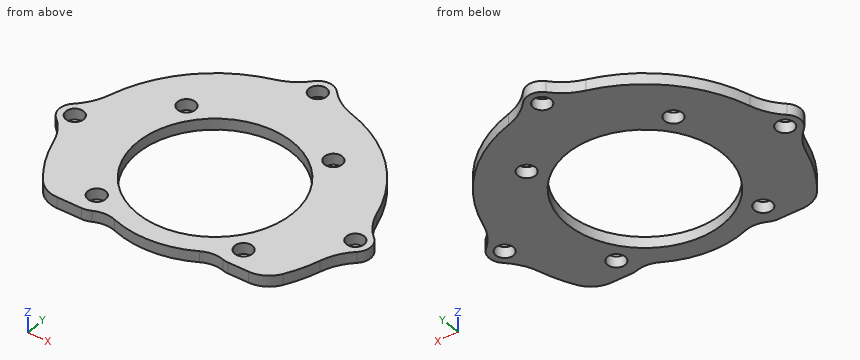
from build123d import *

# Parameters (mm, degrees)
SKETCH1_R           = 25
SKETCH1_R_2         = 3
BOSS_EXTRUDE1_DEPTH = 2
FILLET1_R           = 10
CUT_EXTRUDE1_DEPTH  = 3.0000001
SKETCH4_R           = 1.6
SKETCH4_R_2         = 14
CUT_EXTRUDE2_DEPTH  = 3.0000001
SKETCH6_R           = 1.6
CUT_EXTRUDE3_DEPTH  = 3.0000001
SKETCH7_OUTSIDE_W   = 73.426
SKETCH7_OUTSIDE_H   = 70.426
CUT_EXTRUDE4_DEPTH  = 10
CUT_EXTRUDE5_DEPTH  = 10
FILLET2_R           = 5


with BuildPart() as part:
    # Sketch1 → Boss-Extrude1 (new body)
    with BuildSketch(Plane.XY):
        with Locations((-25, -40.1)):
            Circle(SKETCH1_R)
        with Locations((-50, -40.1)):
            Circle(SKETCH1_R_2)
        with Locations((-50, -40.1)):
            Circle(SKETCH1_R_2)
        with Locations((-25, -40.1)):
            Circle(SKETCH1_R)
        with Locations((0, -40.1)):
            Circle(SKETCH1_R_2)
        with Locations((-25, -40.1)):
            Circle(SKETCH1_R)
        with Locations((-25, -15.1)):
            Circle(SKETCH1_R_2)
        with Locations((-50, -40.1)):
            Circle(SKETCH1_R_2)
        with Locations((-25, -40.1)):
            Circle(SKETCH1_R)
        with Locations((-25, -15.1)):
            Circle(SKETCH1_R_2)
        with Locations((-25, -15.1)):
            Circle(SKETCH1_R_2)
        with Locations((-25, -40.1)):
            Circle(SKETCH1_R)
        with Locations((-25, -40.1)):
            Circle(SKETCH1_R)
        with Locations((0, -40.1)):
            Circle(SKETCH1_R_2)
        with Locations((0, -40.1)):
            Circle(SKETCH1_R_2)
        with Locations((-25, -40.1)):
            Circle(SKETCH1_R)
    extrude(amount=BOSS_EXTRUDE1_DEPTH)

    # Fillet1
    fillet1_edges = [part.edges().sort_by_distance(p)[0] for p in [
        (-49.82, -37.105404869, 1),
        (-27.994595131, -15.28, 1),
        (-22.005404869, -15.28, 1),
        (-0.18, -37.105404869, 1),
        (-0.18, -43.094595131, 1),
        (-49.82, -43.094595131, 1),
    ]]
    fillet(fillet1_edges, radius=FILLET1_R)

    # Sketch3 → Cut-Extrude1 (cut, through all)
    with BuildSketch(Plane.XY.offset(2)):
        with BuildLine():
            ThreePointArc((-37.216735292, -29.767928139), (-37.401620542, -27.65468006), (-39.514868621, -27.83956531))
            ThreePointArc((-39.514868621, -27.83956531), (-39.329983371, -29.952813389), (-37.216735292, -29.767928139))
        make_face()
        with BuildLine():
            ThreePointArc((-35.332071861, -52.316735292), (-37.44531994, -52.501620542), (-37.26043469, -54.614868621))
            ThreePointArc((-37.26043469, -54.614868621), (-35.147186611, -54.429983371), (-35.332071861, -52.316735292))
        make_face()
        with BuildLine():
            ThreePointArc((-12.783264708, -50.432071861), (-12.598379458, -52.54531994), (-10.485131379, -52.36043469))
            ThreePointArc((-10.485131379, -52.36043469), (-10.670016629, -50.247186611), (-12.783264708, -50.432071861))
        make_face()
        with BuildLine():
            ThreePointArc((-14.667928139, -27.883264708), (-12.55468006, -27.698379458), (-12.73956531, -25.585131379))
            ThreePointArc((-12.73956531, -25.585131379), (-14.852813389, -25.770016629), (-14.667928139, -27.883264708))
        make_face()
        with BuildLine():
            ThreePointArc((-35.264995538, -31.48664603), (-33.61335397, -50.364995538), (-14.735004462, -48.71335397))
            ThreePointArc((-14.735004462, -48.71335397), (-16.38664603, -29.835004462), (-35.264995538, -31.48664603))
        make_face()
    extrude(amount=-CUT_EXTRUDE1_DEPTH, mode=Mode.SUBTRACT)

    # Sketch4 → Cut-Extrude2 (cut, through all)
    with BuildSketch(Plane.XY.offset(2)):
        with Locations((-36.296253275, -53.465801956)):
            Circle(SKETCH4_R)
        with Locations((-38.365801956, -28.803746725)):
            Circle(SKETCH4_R)
        with Locations((-13.703746725, -26.734198044)):
            Circle(SKETCH4_R)
        with Locations((-11.634198044, -51.396253275)):
            Circle(SKETCH4_R)
        with Locations((-25, -40.1)):
            Circle(SKETCH4_R_2)
    extrude(amount=-CUT_EXTRUDE2_DEPTH, mode=Mode.SUBTRACT)

    # Sketch6 → Cut-Extrude3 (cut, through all)
    with BuildSketch(Plane.XY.offset(2)):
        with Locations((-50, -40.1)):
            Circle(SKETCH6_R)
        with Locations((-25, -15.1)):
            Circle(SKETCH6_R)
        with Locations((0, -40.1)):
            Circle(SKETCH6_R)
    extrude(amount=-CUT_EXTRUDE3_DEPTH, mode=Mode.SUBTRACT)

    # Sketch7 outside → Cut-Extrude4 (cut)
    with BuildSketch(Plane.XY.offset(2)):
        with Locations((-25, -38.6)):
            Rectangle(SKETCH7_OUTSIDE_W, SKETCH7_OUTSIDE_H)
        with BuildLine():
            ThreePointArc((-31.881324829, -16.325857143), (-42.500892834, -22.599107166), (-48.774142857, -33.218675171))
            ThreePointArc((-48.774142857, -33.218675171), (-49.956443907, -35.846542569), (-51.823461538, -38.041484025))
            ThreePointArc((-51.823461538, -38.041484025), (-52.75, -40.1), (-51.823461538, -42.158515975))
            ThreePointArc((-51.823461538, -42.158515975), (-49.956443907, -44.353457431), (-48.774142857, -46.981324829))
            ThreePointArc((-48.774142857, -46.981324829), (-25, -64.85), (-1.225857143, -46.981324829))
            ThreePointArc((-1.225857143, -46.981324829), (-0.043556093, -44.353457431), (1.823461538, -42.158515975))
            ThreePointArc((1.823461538, -42.158515975), (2.75, -40.1), (1.823461538, -38.041484025))
            ThreePointArc((1.823461538, -38.041484025), (-0.043556093, -35.846542569), (-1.225857143, -33.218675171))
            ThreePointArc((-1.225857143, -33.218675171), (-7.499107166, -22.599107166), (-18.118675171, -16.325857143))
            ThreePointArc((-18.118675171, -16.325857143), (-20.746542569, -15.143556093), (-22.941484025, -13.276538462))
            ThreePointArc((-22.941484025, -13.276538462), (-25, -12.35), (-27.058515975, -13.276538462))
            ThreePointArc((-27.058515975, -13.276538462), (-29.253457431, -15.143556093), (-31.881324829, -16.325857143))
        make_face(mode=Mode.SUBTRACT)
    extrude(amount=-CUT_EXTRUDE4_DEPTH, mode=Mode.SUBTRACT)

    # Sketch8 → Cut-Extrude5 (cut)
    with BuildSketch(Plane.XY.offset(2)):
        with BuildLine():
            ThreePointArc((-33.189286906, -55.565625754), (-34.537253452, -56.777662403), (-36.296253275, -57.215801956))
            Line((-36.296253275, -57.215801956), (-42.877690662, -57.215801956))
            ThreePointArc((-42.877690662, -57.215801956), (-23.637222782, -64.812453101), (-5.348721101, -55.146253275))
            Line((-5.348721101, -55.146253275), (-11.634198044, -55.146253275))
            ThreePointArc((-11.634198044, -55.146253275), (-13.110091293, -54.843605755), (-14.347757645, -53.984514137))
            ThreePointArc((-14.347757645, -53.984514137), (-23.536608094, -57.538706492), (-33.189286906, -55.565625754))
        make_face()
    extrude(amount=-CUT_EXTRUDE5_DEPTH, mode=Mode.SUBTRACT)

    # Fillet2
    fillet2_edges = [part.edges().sort_by_distance(p)[0] for p in [
        (-42.877690662, -57.215801956, 1),
        (-5.348721101, -55.146253275, 1),
        (-14.347757645, -53.984514137, 1),
        (-33.189286906, -55.565625754, 1),
    ]]
    fillet(fillet2_edges, radius=FILLET2_R)


solid = part.part
CAD build for the part. Positions are in the model's coordinates, mm. Give positions to 0.01 mm unless a question says otherwise; leave off trailing zeros. Write each loop counter-clockwise with the first axis right and the second up, starting at its lowest first coordinate (ties: lowest second). Pieces come first, ordered by that corner, then holes. Notation, with made-up numbers: (-23.5, 70.5) - (8.5, 70.5) arc R28 ccw to (8.5, 93.5) - close; hole circle Ø4 at (62, 41). An arc over 180 degrees is marked (long way). Put each result on its own line as item: value.
(1) Wall check: L1, parallel to Y at x = -25, z = 0.9; L2, parallel to Y at x = -24, z = 1.9; L3, parallel to X at y = -49.5, z = 0.7. Give the ranges that are in metal, low to high.
Working result:
L1: -57.6 to -54.1, -26.1 to -16.7, -13.5 to -12.35
L2: -57.57 to -54.06, -26.14 to -16.35, -13.85 to -12.54
L3: -47.9 to -35.37, -14.63 to -2.1
(2) Saw through at C-C (x = 0). List the corners of the cut face in (y, z), then the cut area to 3 significant figures.
Working result:
outline: (-44.29, 0) - (-41.7, 0) - (-41.7, 2) - (-44.29, 2) - close; (-38.5, 0) - (-35.91, 0) - (-35.91, 2) - (-38.5, 2) - close
area: 10.3 mm^2
(3) Saw through at D-D (y = -15.1). List the corners of the cut face in (x, z), then the cut area to 3 significant figures.
Working result:
outline: (-29.19, 0) - (-26.6, 0) - (-26.6, 2) - (-29.19, 2) - close; (-23.4, 0) - (-20.81, 0) - (-20.81, 2) - (-23.4, 2) - close
area: 10.3 mm^2
(4) Saw through at A-A (y = -40.1). List the corners of the cut face in (x, z), then the cut area to 3 significant figures.
Working result:
outline: (-52.75, 0) - (-51.6, 0) - (-51.6, 2) - (-52.75, 2) - close; (-48.4, 0) - (-39, 0) - (-39, 2) - (-48.4, 2) - close; (-11, 0) - (-1.6, 0) - (-1.6, 2) - (-11, 2) - close; (1.6, 0) - (2.75, 0) - (2.75, 2) - (1.6, 2) - close
area: 42.2 mm^2
(5) Drop flat-ended pins along their axis: pin 1 Ø3.5 at (x, y) = (-11.63, -51.4) entering from -Z; pin 2 Ø1 at (y, z) = (-35, 1.5) entering from -X. Give the stop position or say it passes through.
Working result:
pin 1: z = 0
pin 2: x = -49.75
(6) Saw through at B-B (x = -25). List the corners of the cut face in (y, z), then the cut area to 3 significant figures.
Working result:
outline: (-57.6, 0) - (-54.1, 0) - (-54.1, 2) - (-57.6, 2) - close; (-26.1, 0) - (-16.7, 0) - (-16.7, 2) - (-26.1, 2) - close; (-13.5, 0) - (-12.35, 0) - (-12.35, 2) - (-13.5, 2) - close
area: 28.1 mm^2
